```python
from build123d import *

# Parameters (mm, degrees)
SKETCH_1_R      = 1.5
EXTRUDE_1_DEPTH = 1.5
EXTRUDE_2_DEPTH = 5.5
SKETCH_3_W      = 4.5
SKETCH_3_H      = 16
EXTRUDE_3_DEPTH = 6
FILLET_1_R      = 2


with BuildPart() as part:
    # Эскиз1 → Бобышка-Вытянуть1 (new body)
    with BuildSketch(Plane(origin=(0, 0, 0), x_dir=(1, 0, 0), z_dir=(0, 1, 0))):
        with BuildLine():
            Line((-28.198313686, 2.834587413), (-28.198313686, -13.165412587))
            ThreePointArc((-28.198313686, -13.165412587), (-27.31963403, -15.286732931), (-25.198313686, -16.165412587))
            Line((-25.198313686, -16.165412587), (-1.198313686, -16.165412587))
            ThreePointArc((-1.198313686, -16.165412587), (0.923006657, -15.286732931), (1.801686314, -13.165412587))
            Line((1.801686314, -13.165412587), (1.801686314, 2.834587413))
            ThreePointArc((1.801686314, 2.834587413), (0.923006657, 4.955907756), (-1.198313686, 5.834587413))
            Line((-1.198313686, 5.834587413), (-25.198313686, 5.834587413))
            ThreePointArc((-25.198313686, 5.834587413), (-27.31963403, 4.955907756), (-28.198313686, 2.834587413))
        make_face()
        with Locations(Location((-25.198313686, -13.165412587, 0), (0, 0, 270))):
            Circle(SKETCH_1_R, mode=Mode.SUBTRACT)
        with Locations(Location((-25.198313686, 2.834587413, 0), (0, 0, 270))):
            Circle(SKETCH_1_R, mode=Mode.SUBTRACT)
    extrude(amount=EXTRUDE_1_DEPTH)

    # Эскиз2 → Бобышка-Вытянуть2 (add)
    with BuildSketch(Plane(origin=(0, 1.5, 0), x_dir=(1, 0, 0), z_dir=(0, 1, 0))):
        Polygon((1.801686314, -0.165412587), (-6.698313686, -0.165412587), (-6.698313686, -10.165412587), (1.801686314, -10.165412587), (3.801686314, -10.165412587), (3.801686314, -0.165412587), align=None)
    extrude(amount=EXTRUDE_2_DEPTH)

    # Эскиз3 → Бобышка-Вытянуть3 (add)
    with BuildSketch(Plane(origin=(0, 1.5, 0), x_dir=(1, 0, 0), z_dir=(0, 1, 0))):
        with Locations((-15.448313686, -5.165412587)):
            Rectangle(SKETCH_3_W, SKETCH_3_H)
    extrude(amount=EXTRUDE_3_DEPTH)

    # Скругление1
    fillet_1_edges = [part.edges().sort_by_distance(p)[0] for p in [
        (-17.698313686, 7.5, 5.165412587),
        (-13.198313686, 7.5, 5.165412587),
    ]]
    fillet(fillet_1_edges, radius=FILLET_1_R)


solid = part.part
```
Here's how the part is built. I have some questions about the finished solid (model axes, mm). A direction names the side the tool comes from. Round coordinates to 2 decimals unless told otherwise and drop trailing zeros. Loops run counter-clockwise (first coordinate to the right, second up) from the corner with the lowest first, then second, coordinate; pieces in that order, holes last. Notation, with made-up numbers: (1, 24.25) -> (31, 24.25) arc R18 cw to (31, 42.25) -> close; hole circle Ø5 at (-28.75, 5). An arc over 180 degrees is marked (long way). Answer as CSV lines item,"result". Start each with the question number.
1. Imagine slicing it at C-C on z = 14. Write out the boundary of the cut face in (x, y).
2. Imagine slicing it at D-D on z = -0.75. Write out the boundary of the cut face in (x, y).
3. For faces 1 (the face through (-2, 4, 10.165)), 2 (the face through (-1, 4, 0.165)), 3 (the face through (1.802, 1, 5)), 4 (the face through (-13.198, 3, 5)), 5 (the face through (-2, 7, 5)), which set-ups out of +Z, -Z, +X, -X, +Y, -Y let a thin tool reach every point of the face, with its end or its side?
4. Imagine slicing it at A-A on y = 2.5. Write out the boundary of the cut face in (x, z), plus the area to 3 significant figures.
5. I'm going to push flat-ended pins straight in: P1, Ø1.6, axis at x = -1.5, y = 3.5, coming from the +Z side; P2, Ø1.6, axis at x = 1, y = 4.5, coming from the -Z side; P3, Ø8, axis at x = 1, z = 4, coming from the +Y side; P4, Ø2.5, axis at x = -25.2, z = -2.83, coming from the +Y side. Where does each tip first touch, or does it pass through?
6. If we mould it in two halves opening along Z, with no side actions, what happens to faces 6 (the face through (-28.198, 1, 5)), 7 (the face through (-26.663, 0.74, -3.16)), 8 (the face through (-27.296, 0.74, -4.979))? For each: pulls with the +Z half, pulls with the -Z half, needs draft (parallel to the pull), parting line crosses it, or undercut.
7. Imagine slicing it at B-B on y = 0.5. Write out the boundary of the cut face in (x, z).
8. I need wall thicknesses on probe 1 along X at (y, z) = (3.5, 5); probe 2 along Y at (x, z) = (-6.5, 14.25); probe 3 along X at (y, z) = (5.5, 12). Which ranges of each line are inside material? Lowest first, please. Write a range as from..to.
Solution:
1,outline,"(-28.08, 0) -> (-26.44, 0) -> (-26.44, 1.5) -> (-28.08, 1.5) -> close; (-23.95, 0) -> (1.68, 0) -> (1.68, 1.5) -> (-23.95, 1.5) -> close"
2,outline,"(-28.2, 0) -> (1.8, 0) -> (1.8, 1.5) -> (-13.2, 1.5) -> (-13.2, 5.5) arc R2 ccw to (-15.2, 7.5) -> (-15.7, 7.5) arc R2 ccw to (-17.7, 5.5) -> (-17.7, 1.5) -> (-28.2, 1.5) -> close"
3,face 1,"+Z, +X, +Y"
3,face 2,"-Z, +X, +Y"
3,face 3,"+Z, -Z, +X, -Y"
3,face 4,"+Z, -Z, +Y"
3,face 5,"+Z, -Z, +X, +Y"
4,outline,"(-17.7, -2.83) -> (-13.2, -2.83) -> (-13.2, 13.17) -> (-17.7, 13.17) -> close; (-6.7, 0.17) -> (3.8, 0.17) -> (3.8, 10.17) -> (-6.7, 10.17) -> close"
4,area,"177 mm²"
5,P1,"z = 10.17"
5,P2,"z = 0.17"
5,P3,"y = 7"
5,P4,"through"
6,face 6,"needs draft"
6,face 7,"undercut"
6,face 8,"pulls with the -Z half"
7,outline,"(-28.2, -2.83) arc R3 ccw to (-25.2, -5.83) -> (-1.2, -5.83) arc R3 ccw to (1.8, -2.83) -> (1.8, 13.17) arc R3 ccw to (-1.2, 16.17) -> (-25.2, 16.17) arc R3 ccw to (-28.2, 13.17) -> close; hole circle Ø3 at (-25.2, -2.83); hole circle Ø3 at (-25.2, 13.17)"
8,probe 1,"-17.7..-13.2, -6.7..3.8"
8,probe 2,"0..1.5"
8,probe 3,"-17.7..-13.2"
